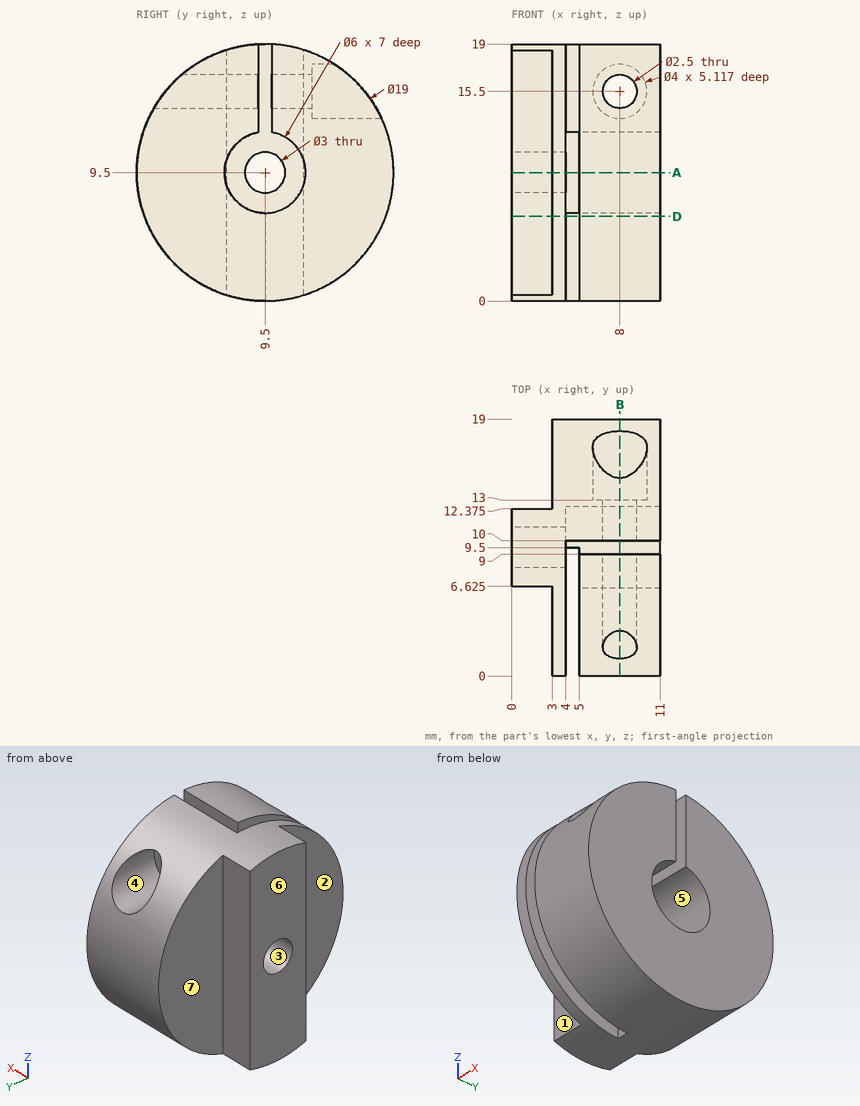
Print and shaded views of the part. All mm, measured from the part's lowest x, y and z. A direction names the side the tool comes from. Round coordinates to 2 decimals unless told otherwise and drop trailing zeros. Write each loop counter-clockwise with the first axis right and the second up, starting at its lowest first coordinate (ties: lowest second). Pieces come first, ordered by that corner, then holes.
Item 1: Probe L1, parallel to X at y = 5, z = 4.25; L2, parallel to X at y = 11.65, z = 15.5; L3, parallel to Y at x = 1.2, z = 9.5 (3 decimals). List the from-to ranges inside material, lowest first.
Results:
L1: x = 3 to 4, 5 to 11
L2: x = 0 to 6.75, 9.25 to 11
L3: y = 6.625 to 8, 11 to 12.375
Item 2: Two-plate mould, pull along Y, no slides. Class the marked faces 1, 2 and 3: +Y half, -Y half, draft (parallel to the pull), parting line (faces both ways), or undercut.
Results:
face 1: -Y half
face 2: draft
face 3: undercut
Item 3: Drop flat-ended pins along their axis: pin 1 Ø6 at (x, y) = (2.5, 4.5) entering from -Z; pin 2 Ø3 at (y, z) = (2, 17) entering from -X; pin 3 Ø2 at (x, z) = (8, 15) entering from +Y; pin 4 Ø2 at (x, z) = (8, 15.5) entering from +Y. Give the stop position or say it passes through.
Results:
pin 1: stops at z = 0.21
pin 2: stops at x = 3
pin 3: stops at y = 13
pin 4: passes through
Item 4: Cut at D-D, the plane z = 6.25. Give the cut face in (x, y) (1 decimal).
Results:
outline: (0, 6.6) - (3, 6.6) - (3, 0.6) - (4, 0.6) - (4, 9.5) - (5, 9.5) - (5, 0.6) - (11, 0.6) - (11, 18.4) - (3, 18.4) - (3, 12.4) - (0, 12.4) - close
Item 5: Cut at B-B, the plane x = 8. Give the cut face in (y, z).
Results:
outline: (1.27, 14.25) arc R9.5 ccw (long way) to (18.12, 13.5) - (13, 13.5) - (13, 14.25) - (10, 14.25) - (10, 12.46) arc R3 cw (long way) to (9, 12.46) - (9, 14.25) - close; (3.36, 16.75) - (9, 16.75) - (9, 18.99) arc R9.5 ccw to start; (10, 16.75) - (13, 16.75) - (13, 17.5) - (14.62, 17.5) arc R9.5 ccw to (10, 18.99) - close
Item 6: Which spindle directions (+Z, -Z, +X, -X, +Y, -Y) get a long thin tool onto all of the face, cutting with end or side? Do the marked faces 4, 5, 6 and 7. Say none if no direction does.
Results:
face 4: +Y
face 5: +X
face 6: +Z, -Z, -X, +Y, -Y
face 7: +Z, -Z, -X, +Y
Item 7: Cut at A-A, the plane z = 9.5. Give the cut face in (x, y) (3 decimals), plus the area to 3 significant figures.
Results:
outline: (0, 6.625) - (3, 6.625) - (3, 0) - (4, 0) - (4, 8) - (0, 8) - close; (0, 11) - (4, 11) - (4, 12.5) - (11, 12.5) - (11, 19) - (3, 19) - (3, 12.375) - (0, 12.375) - close; (5, 0) - (11, 0) - (11, 6.5) - (5, 6.5) - close
area: 109 mm2
